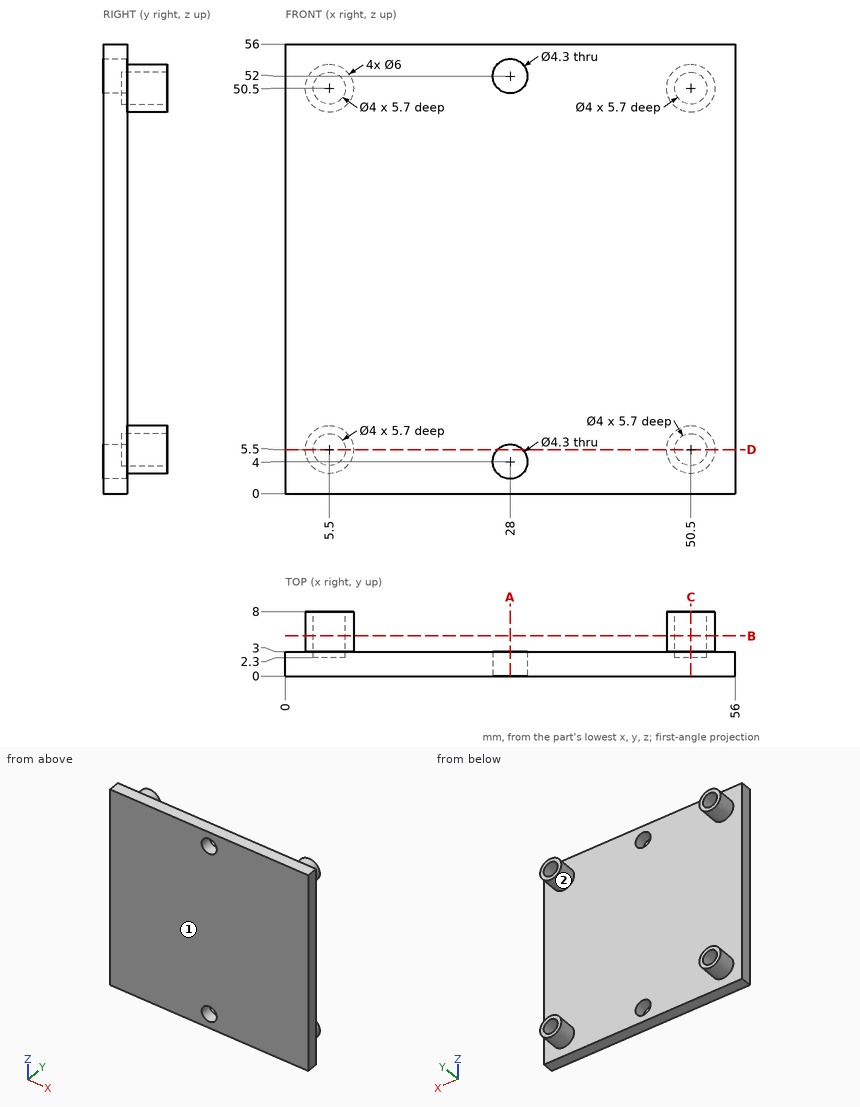
The figure shows three views and two pictorial views of one solid part (mm, origin at its lowest corner). Answer the questions. Give positions to 0.01 mm unless a question says otherwise; leave off trailing zeros. Order: outer loops, then holes, each group sorted by start corner. A loop starts at its lowest first (then second) coordinate and runs counter-clockwise, first axis right, second up. Notation, with made-up numbers: (-1, 6) -> (14, 6) arc R13 cw to (14, 21) -> close; hole circle Ø3 at (50.25, 22.25). An arc over 180 degrees is marked (long way). Answer as CSV lines item,"result". Start each with the question number.
(1) Consider line 1 along X through (y, z) = (5.6, 5.5); line 2 along Y through (x, z) = (38.5, 14.5); line 3 along Z through (x, y) = (50, 7.75). Determine where each line is inside the solid, lowest interval first.
(2) For a pull along X with two mould halves and no side action, classify the marked faces 1 and 2 as released by +X, released by -X, zero draft, split by the parting line, or undercut.
(3) Section D-D, the plane z = 5.5 is taken. Write down the section's boundary in (x, y).
(4) Section A-A, the plane x = 28 is taken. Write down the section's boundary in (y, z), plus the area to 3 significant figures.
(5) Each of these flat-tipped pins is pushed along its axis until it touches: pin 1 Ø4.5 at (x, z) = (50.5, 50.5) entering from -Y; pin 2 Ø3.5 at (x, z) = (28, 4) entering from +Y; pin 3 Ø1.2 at (x, z) = (5, 51) entering from +Y. Where does it stop, or does it pass through?
(6) Section B-B, the plane y = 5 is taken. Write down the section's boundary in (x, z), plus the area to 3 significant figures.
(7) Section C-C, the plane x = 50.5 is taken. Write down the section's boundary in (y, z), plus the area to 3 significant figures.
Entries:
1,line 1,"2.5 to 3.5, 7.5 to 8.5, 47.5 to 48.5, 52.5 to 53.5"
1,line 2,"0 to 3"
1,line 3,"2.54 to 3.56, 7.44 to 8.46, 47.54 to 48.56, 52.44 to 53.46"
2,face 1,"zero draft"
2,face 2,"undercut"
3,outline,"(0, 0) -> (26.46, 0) -> (26.46, 3) -> (8.5, 3) -> (8.5, 8) -> (7.5, 8) -> (7.5, 2.3) -> (3.5, 2.3) -> (3.5, 8) -> (2.5, 8) -> (2.5, 3) -> (0, 3) -> close; (29.54, 0) -> (56, 0) -> (56, 3) -> (53.5, 3) -> (53.5, 8) -> (52.5, 8) -> (52.5, 2.3) -> (48.5, 2.3) -> (48.5, 8) -> (47.5, 8) -> (47.5, 3) -> (29.54, 3) -> close"
4,outline,"(0, 0) -> (3, 0) -> (3, 1.85) -> (0, 1.85) -> close; (0, 6.15) -> (3, 6.15) -> (3, 49.85) -> (0, 49.85) -> close; (0, 54.15) -> (3, 54.15) -> (3, 56) -> (0, 56) -> close"
4,area,"142 mm²"
5,pin 1,"y = 0"
5,pin 2,"through"
5,pin 3,"y = 2.3"
6,outline,"circle Ø6 at (5.5, 5.5); circle Ø6 at (5.5, 50.5); circle Ø6 at (50.5, 5.5); circle Ø6 at (50.5, 50.5); hole circle Ø4 at (5.5, 5.5); hole circle Ø4 at (5.5, 50.5); hole circle Ø4 at (50.5, 5.5); hole circle Ø4 at (50.5, 50.5)"
6,area,"62.8 mm²"
7,outline,"(0, 0) -> (3, 0) -> (3, 2.5) -> (8, 2.5) -> (8, 3.5) -> (2.3, 3.5) -> (2.3, 7.5) -> (8, 7.5) -> (8, 8.5) -> (3, 8.5) -> (3, 47.5) -> (8, 47.5) -> (8, 48.5) -> (2.3, 48.5) -> (2.3, 52.5) -> (8, 52.5) -> (8, 53.5) -> (3, 53.5) -> (3, 56) -> (0, 56) -> close"
7,area,"182 mm²"
